Build history of the part. All positions in model axes, mm. Face numbers are marked on the shaded views. A direction names the side the tool comes from. Give positions to 0.01 mm unless a question says otherwise; leave off trailing zeros. Order: outer loops, then holes, each group sorted by start corner. A loop starts at its lowest first (then second) coordinate and runs counter-clockwise, first axis right, second up. Notation, with made-up numbers: (13.25, -34) - (64.25, -34) arc R12 cw to (64.25, -21) - close; hole circle Ø7 at (48.5, 19.5). An arc over 180 degrees is marked (long way). One line per item, written item: value.
```python
from build123d import *

# Parameters (mm, degrees)
SKETCH_W        = 20
SKETCH_H        = 20
PAD_DEPTH       = 30
PAD001_DEPTH    = 20
SKETCH002_W     = 13
SKETCH002_H     = 16
POCKET_DEPTH    = 27
SKETCH003_R     = 3
POCKET001_DEPTH = 8.001
SKETCH004_R     = 6
POCKET002_DEPTH = 1
CHAMFER_SIZE    = 2.5
FILLET_R        = 4
FILLET001_R     = 1
FILLET002_R     = 6
SKETCH005_R     = 3.25
POCKET003_DEPTH = 5


with BuildPart() as part:
    # Sketch → Pad (new body)
    with BuildSketch(Plane.XY):
        Rectangle(SKETCH_W, SKETCH_H)
    extrude(amount=PAD_DEPTH)

    # Sketch001 (on Face1 of Pad) → Pad001 (join)
    with BuildSketch(Plane(origin=(0, 10, 0), x_dir=(-1, 0, 0), z_dir=(0, 1, 0))):
        Polygon((10, 25.8), (10, 20), (10, 14.2), (11, 14.2), (11, 25.8), align=None)
    extrude(amount=-PAD001_DEPTH)

    # Sketch002 (on Face7 of Pad001) → Pocket (cut)
    with BuildSketch(Plane.XY.offset(30)):
        with Locations((3.5, -2)):
            Rectangle(SKETCH002_W, SKETCH002_H)
    extrude(amount=-POCKET_DEPTH, mode=Mode.SUBTRACT)

    # Sketch003 (on Face12 of Pocket) → Pocket001 (cut, through all)
    with BuildSketch(Plane.YZ.offset(-3)):
        with Locations((-2, 20)):
            Circle(SKETCH003_R)
    extrude(amount=-POCKET001_DEPTH, mode=Mode.SUBTRACT)

    # Sketch004 (on Face12 of Pocket001) → Pocket002 (cut)
    with BuildSketch(Plane.YZ.offset(-3)):
        with Locations((-2, 20)):
            Circle(SKETCH004_R)
    extrude(amount=-POCKET002_DEPTH, mode=Mode.SUBTRACT)

    # Chamfer
    chamfer_edges = [part.edges().sort_by_distance(p)[0] for p in [
        (-4, -5, 20),
    ]]
    chamfer(chamfer_edges, length=CHAMFER_SIZE)

    # Fillet
    fillet_edges = [part.edges().sort_by_distance(p)[0] for p in [
        (-6.5, -10, 30),
    ]]
    fillet(fillet_edges, radius=FILLET_R)

    # Fillet001
    fillet001_edges = [part.edges().sort_by_distance(p)[0] for p in [
        (-3, -10, 14.5),
        (-3, 6, 16.5),
        (-3, -2, 3),
        (3.5, 6, 3),
    ]]
    fillet(fillet001_edges, radius=FILLET001_R)

    # Fillet002
    fillet002_edges = [part.edges().sort_by_distance(p)[0] for p in [
        (10, -10, 1.5),
        (10, 8, 30),
    ]]
    fillet(fillet002_edges, radius=FILLET002_R)

    # Sketch005 (on Face2 of Fillet002) → Pocket003 (cut)
    with BuildSketch(Plane(origin=(0, 10, 0), x_dir=(-1, 0, 0), z_dir=(0, 1, 0))):
        with Locations((-3, 10)):
            Circle(SKETCH005_R)
    extrude(amount=-POCKET003_DEPTH, mode=Mode.SUBTRACT)


solid = part.part
```
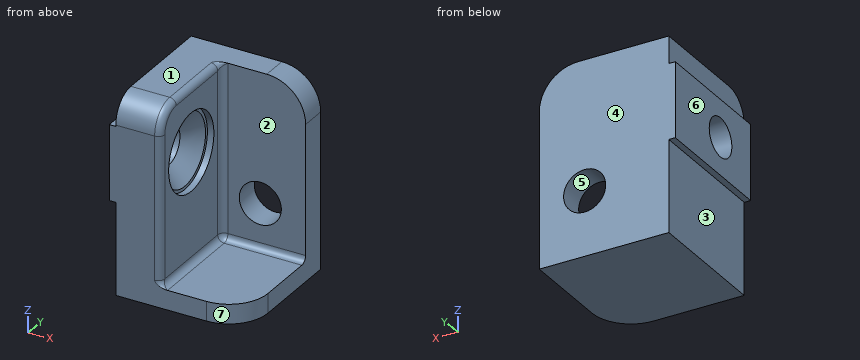
(1) 3-axis set-ups, long thin cutter, end or side, ignore diameter. For the marked faces 1, 2 and 3: which of +Z, -Z, +X, -X, +Y, -Y reach the whole face in a straight line?
Completed:
face 1: +Z, +X, -X, +Y, -Y
face 2: +Z, +X, -Y
face 3: -Z, -X, +Y, -Y
(2) Drill centre lines: line 1 (Z direction, x = 3, y = 8.3); line 2 (Z direction, x = -10.1, y = -2); line 3 (X direction, y = -7.5, z = 12). Where is each one in solid material? Low to high.
Completed:
line 1: 0 to 6.75, 13.25 to 30
line 2: 14.2 to 17, 23 to 25.8
line 3: -10 to -3
(3) Slice it at D-D, the plane x = -5.75. Give the cut face in (y, z).
Completed:
outline: (-10, 0) - (10, 0) - (10, 30) - (-6, 30) arc R4 ccw to (-10, 26) - close; hole circle Ø7.5 at (-2, 20)
(4) Slice it at C-C, the plane x = 3. Give the cut face in (y, z).
Completed:
outline: (-10, 0) - (10, 0) - (10, 6.75) - (6, 6.75) - (6, 4) arc R1 cw to (5, 3) - (-10, 3) - close; (6, 13.25) - (10, 13.25) - (10, 30) - (6, 30) - close
(5) Pin check, flat tips, straight feed: P1, Ø4, axis at y = 1.5, z = 11, coming from the -X side; P2, Ø1, axis at x = -3.5, y = 0.5, coming from the +Z side; P3, Ø2, axis at x = -0.5, z = 19.5, coming from the -Y side; P4, Ø3.5, axis at x = 3, y = 0, coming from the +Z side. Stop position of each tip, or through.
Completed:
P1: x = -10
P2: z = 30
P3: y = 6
P4: z = 3
(6) Slice it at B-B, the plane y = -2. Give the cut face in (x, z).
Completed:
outline: (-11, 14.2) - (-10, 14.2) - (-10, 0) - (10, 0) - (10, 3) - (-2, 3) arc R1 cw to (-3, 4) - (-3, 14) - (-4, 14) - (-4, 14.5) - (-6.5, 17) - (-11, 17) - close; (-11, 23) - (-6.5, 23) - (-4, 25.5) - (-4, 26) - (-3, 26) - (-3, 29) arc R1 ccw to (-4, 30) - (-10, 30) - (-10, 25.8) - (-11, 25.8) - close
(7) Slice it at A-A, the plane z = 20. Give the cut face in (x, y), and give its area (3 significant figures).
Completed:
outline: (-11, -10) - (-4, -10) arc R1 ccw to (-3, -9) - (-3, -8) - (-4, -8) - (-4, -7.5) - (-6.5, -5) - (-11, -5) - close; (-11, 1) - (-6.5, 1) - (-4, 3.5) - (-4, 4) - (-3, 4) - (-3, 5) arc R1 cw to (-2, 6) - (10, 6) - (10, 10) - (-11, 10) - close
area: 152 mm²
(8) Pull direction X, two halves, no side cores. Call the marked faces 4, 5, 6 and 7: +X half, -X half, draft (parallel to the pull), parting line (faces both ways), or undercut.
Completed:
face 4: draft
face 5: undercut
face 6: -X half
face 7: +X half
